from build123d import *

# Parameters (mm, degrees)
F1_DEPTH = 3.175
F2_W     = 25.4
F2_H     = 88.9
F3_DEPTH = 7.9375


with BuildPart() as f1:
    # F0 (on Front) → F1 (new body, symmetric)
    with BuildSketch(Plane.XZ):
        with BuildLine():
            Line((-12.7, 88.9), (-12.7, 0))
            Line((-12.7, 0), (12.7, 0))
            Line((12.7, 0), (12.7, 88.9))
            ThreePointArc((12.7, 88.9), (0, 240.234213), (-12.7, 88.9))
        make_face()
    extrude(amount=F1_DEPTH, both=True)

    # F2 (on face) → F3 (join)
    with BuildSketch(Plane.XZ.offset(3.175)):
        with Locations((0, 44.45)):
            Rectangle(F2_W, F2_H)
    extrude(amount=F3_DEPTH)


solid = f1.part
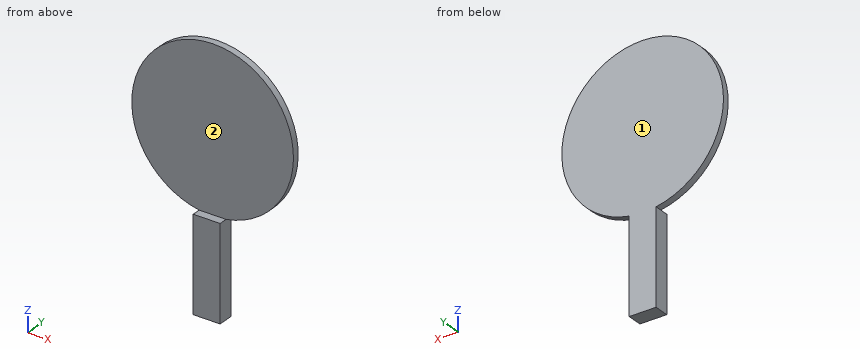
CAD build for the part. Positions are in the model's coordinates, mm. Face numbers are marked on the shaded views. A direction names the side the tool comes from. Give positions to 0.01 mm unless a question says otherwise; leave off trailing zeros. Write each loop counter-clockwise with the first axis right and the second up, starting at its lowest first coordinate (ties: lowest second). Pieces come first, ordered by that corner, then holes. Notation, with made-up numbers: M 70,78.25 L 92,78.25 A16 ccw 92,85.25 Z; hole C -40,-17.75 d11. An arc over 180 degrees is marked long. Put each result on its own line as item: value. Start each with the question number.
(1) Probe L1, parallel to Y at x = 5, z = 106.5 (3 decimals); L2, parallel to X at y = -10.25, z = 74; L3, parallel to Z at x = -58, y = -0.75. List the from-to ranges inside material, lowest first.
(2) Band-saw the part on A-A, the plane x = 0. Write the cut outline in (y, z) (1 decimal), and give its area (3 significant figures).
(3) Band-saw the part on C-C, the plane z = 41. Write the cut outline in (x, y) (1 decimal), and give its area (3 significant figures).
(4) Which spindle directions (+Z, -Z, +X, -X, +Y, -Y) get a long thin tool onto all of the face, cutting with end or side? Do the marked faces 1 and 2. Say none if no direction does.
(5) Band-saw the part on B-B, the plane y = -5.75. Write the cut outline in (x, z).
(6) Flat gauge pins, fed straight in: pin 1 Ø1 at (x, y) = (9.5, -6) entering from +Z; pin 2 Ø4.5 at (y, z) = (-3.5, 25) entering from -X; pin 3 Ø3 at (y, z) = (-4.5, 169.5) entering from +X; pin 4 Ø4 at (x, y) = (-1.5, -3) entering from -Z. Where does each tip first touch, or does it go through?
Response values:
1. L1: y = -3.175 to 3.175
1. L2: x = -12.7 to 12.7
1. L3: z = 114.61 to 213.46
2. outline: M -11.1,0 L 3.2,0 L 3.2,240.2 L -3.2,240.2 L -3.2,88.9 L -11.1,88.9 Z
2. area: 2,230 mm2
3. outline: M -12.7,-11.1 L 12.7,-11.1 L 12.7,3.2 L -12.7,3.2 Z
3. area: 363 mm2
4. face 1: +Z, -Z, +X, -X, +Y
4. face 2: +Z, +X, -X, -Y
5. outline: M -12.7,0 L 12.7,0 L 12.7,88.9 L -12.7,88.9 Z
6. pin 1: stops at z = 88.9
6. pin 2: stops at x = -12.7
6. pin 3: stops at x = 76.05
6. pin 4: stops at z = 0
